from build123d import *

# Parameters (mm, degrees)
SKETCH1_R           = 50
BOSS_EXTRUDE1_DEPTH = 5
CUT_EXTRUDE1_DEPTH  = 6
CUT_EXTRUDE2_DEPTH  = 6


with BuildPart() as part:
    # Sketch1 → Boss-Extrude1 (new body)
    with BuildSketch(Plane(origin=(0, 0, 0), x_dir=(1, 0, 0), z_dir=(0, 1, 0))):
        Circle(SKETCH1_R)
    extrude(amount=BOSS_EXTRUDE1_DEPTH)

    # Sketch3 → Cut-Extrude1 (cut, through all)
    with BuildSketch(Plane(origin=(0, 5, 0), x_dir=(1, 0, 0), z_dir=(0, 1, 0))):
        with BuildLine():
            Line((-1, 1.5), (1, 1.5))
            ThreePointArc((1, 1.5), (2.5, 0), (1, -1.5))
            Line((1, -1.5), (-1, -1.5))
            ThreePointArc((-1, -1.5), (-2.5, 0), (-1, 1.5))
        make_face()
    extrude(amount=-CUT_EXTRUDE1_DEPTH, mode=Mode.SUBTRACT)

    # Sketch5 → Cut-Extrude2 (cut, through all)
    with BuildSketch(Plane(origin=(0, 5, 0), x_dir=(1, 0, 0), z_dir=(0, 1, 0))):
        with BuildLine():
            Line((-10, -35), (10, -35))
            ThreePointArc((10, -35), (15, -40), (10, -45))
            Line((10, -45), (-10, -45))
            ThreePointArc((-10, -45), (-15, -40), (-10, -35))
        make_face()
    extrude(amount=-CUT_EXTRUDE2_DEPTH, mode=Mode.SUBTRACT)


solid = part.part
Could you check a few things on this model? Use its own coordinates, in mm. A direction names the side the tool comes from. Round coordinates to 2 decimals unless told otherwise and drop trailing zeros. Loops run counter-clockwise (first coordinate to the right, second up) from the corner with the lowest first, then second, coordinate; pieces in that order, holes last. Notation, with made-up numbers: (-35.75, -34) -> (-5.75, -34) arc R21 ccw to (-5.75, -30) -> close; hole circle Ø8 at (-21.5, 1.25). An arc over 180 degrees is marked (long way). Use CSV: the item, a comma, the result in double quotes.
(1) Suppose I cut it at B-B on y = 2.4. Write out the boundary of the cut face in (x, z).
Return value:
outline,"circle Ø100 at (0, 0); hole (-10, 35) -> (10, 35) arc R5 ccw to (10, 45) -> (-10, 45) arc R5 ccw to start; hole (-1, -1.5) -> (1, -1.5) arc R1.5 ccw to (1, 1.5) -> (-1, 1.5) arc R1.5 ccw to start"
(2) For faces 5 (the flat face through (0, 3, 45)), 6 (the flat face through (10, 0, -1)), which set-ups out of +Z, -Z, +X, -X, +Y, -Y let a thin tool reach every point of the face, with its end or its side?
Return value:
face 5,"+Y, -Y"
face 6,"+Z, -Z, +X, -X, -Y"
(3) Suppose I cut it at C-C on x = 12.5. Write out the boundary of the cut face in (y, z).
Return value:
outline,"(0, -48.41) -> (5, -48.41) -> (5, 35.67) -> (0, 35.67) -> close; (0, 44.33) -> (5, 44.33) -> (5, 48.41) -> (0, 48.41) -> close"
(4) Will these pins go through, and if not, where does the flat tip stop? pin 1 Ø1.5 at (x, y) = (12.5, 3.5) entering from +Z; pin 2 Ø1 at (x, y) = (35, 4.5) entering from +Z; pin 3 Ø1.5 at (x, y) = (27.5, 1.5) entering from -Z.
Return value:
pin 1,"stops at z = 48.6"
pin 2,"stops at z = 36.19"
pin 3,"stops at z = -42.24"
(5) Suppose I cut it at A-A on z = 40. Write out the boundary of the cut face in (x, y).
Return value:
outline,"(-30, 0) -> (-15, 0) -> (-15, 5) -> (-30, 5) -> close; (15, 0) -> (30, 0) -> (30, 5) -> (15, 5) -> close"
(6) Suppose I cut it at D-D on z = 15.5. Write out the boundary of the cut face in (x, y), plus the area to 3 significant figures.
Return value:
outline,"(-47.54, 0) -> (47.54, 0) -> (47.54, 5) -> (-47.54, 5) -> close"
area,"475 mm²"
(7) If we mould it in two halves opening along Z, with no side actions, what happens to faces 1 (the flat face through (0, 3, 35)), 2 (the flat face through (10, 5, -1)), 3 (the cylindrical face through (47.69, 2.46, -15.02)), 4 (the cylindrical face through (-2.5, 2.5, 0))? For each: +Z half, -Z half, draft (parallel to the pull), parting line (faces both ways), or undercut.
Return value:
face 1,"undercut"
face 2,"draft"
face 3,"parting line"
face 4,"undercut"
(8) If I drill on probe 1 along Z at (x, y) = (-1.5, 1.4); probe 2 along X at (y, z) = (3.6, 39); probe 3 along Z at (x, y) = (7, 1.9), over which ranges is the centre line in solid material (lowest first)? Write a range as [from, to].
Return value:
probe 1,"z = [-49.98, -1.41], [1.41, 35], [45, 49.98]"
probe 2,"x = [-31.29, -14.9], [14.9, 31.29]"
probe 3,"z = [-49.51, 35], [45, 49.51]"
